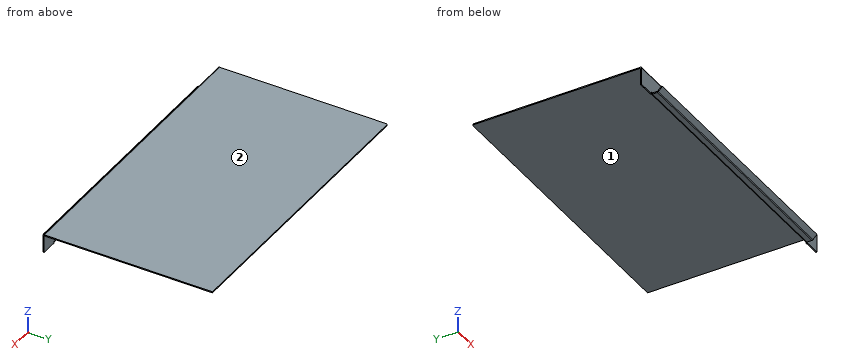
from build123d import *

# Parameters (mm, degrees)
SKETCH_1_W                        = 400
SKETCH_1_H                        = 230
SM_BASE_FLANGE_1_DEPTH            = 1.5
SM_EDGE_FLANGE_1_STRIP_W          = 6.6
SM_EDGE_FLANGE_1_STRIP_H          = 1.5
SM_EDGE_FLANGE_1_STRIP_CUT_DEPTH  = 400
SM_EDGE_FLANGE_1_DEPTH            = 400
SM_EDGE_FLANGE_2_STRIP_W          = 7
SM_EDGE_FLANGE_2_STRIP_H          = 1.5
SM_EDGE_FLANGE_2_STRIP_CUT_DEPTH  = 353
SM_EDGE_FLANGE_2_RELIEF_W         = 7.75
SM_EDGE_FLANGE_2_RELIEF_H         = 0.75
SM_EDGE_FLANGE_2_RELIEF_CUT_DEPTH = 1.5
SM_EDGE_FLANGE_2_DEPTH            = 353
FILLET_1_R                        = 2
SM_START                          = -176.5
SM_EDGE_FLANGE_3_DEPTH            = 353
SM_EDGE_FLANGE_3_2_DEPTH          = 353


# Read off the part's stored shape, not the designer's step: 边线-法兰3
# Sheet-metal steps are written as plain solids
with BuildPart() as part:
    # Sketch 1 → 基体-法兰1 (new body)
    with BuildSketch(Plane.XY):
        Rectangle(SKETCH_1_W, SKETCH_1_H)
    extrude(amount=-SM_BASE_FLANGE_1_DEPTH)

    # 边线-法兰1 strip (across the edge) → 边线-法兰1 strip cut (cut)
    with BuildSketch(Plane(origin=(200, -115, -1.5), x_dir=(0, 1, 0), z_dir=(-1, 0, 0))):
        with Locations((-1.5, -0.75)):
            Rectangle(SM_EDGE_FLANGE_1_STRIP_W, SM_EDGE_FLANGE_1_STRIP_H)
    extrude(amount=SM_EDGE_FLANGE_1_STRIP_CUT_DEPTH, mode=Mode.SUBTRACT)

    # 边线-法兰1 section (across the edge) → 边线-法兰1 (add)
    with BuildSketch(Plane(origin=(200, -115, -1.5), x_dir=(0, 1, 0), z_dir=(-1, 0, 0))):
        with BuildLine():
            Line((0, 0.3), (0, 23.5))
            Line((0, 23.5), (1.5, 23.5))
            Line((1.5, 23.5), (1.5, 0.3))
            ThreePointArc((1.5, 0.3), (1.587867966, 0.087867966), (1.8, 0))
            Line((1.8, 0), (1.8, -1.5))
            ThreePointArc((1.8, -1.5), (0.527207794, -0.972792206), (0, 0.3))
        make_face()
    extrude(amount=SM_EDGE_FLANGE_1_DEPTH)

    # 边线-法兰2 strip (across the edge) → 边线-法兰2 strip cut (cut)
    with BuildSketch(Plane(origin=(-176.5, -115, -25), x_dir=(0, 0, 1), z_dir=(1, 0, 0))):
        with Locations((-1.5, -0.75)):
            Rectangle(SM_EDGE_FLANGE_2_STRIP_W, SM_EDGE_FLANGE_2_STRIP_H)
    extrude(amount=SM_EDGE_FLANGE_2_STRIP_CUT_DEPTH, mode=Mode.SUBTRACT)

    # 边线-法兰2 relief (on the sheet) → 边线-法兰2 relief cut (cut)
    with BuildSketch(Plane(origin=(-176.5, -115, -23), x_dir=(0, 0, 1), z_dir=(0, -1, 0))):
        with Locations((-3.125, 0.375)):
            Rectangle(SM_EDGE_FLANGE_2_RELIEF_W, SM_EDGE_FLANGE_2_RELIEF_H)
        with Locations((-3.125, -353.375)):
            Rectangle(SM_EDGE_FLANGE_2_RELIEF_W, SM_EDGE_FLANGE_2_RELIEF_H)
    extrude(amount=-SM_EDGE_FLANGE_2_RELIEF_CUT_DEPTH, mode=Mode.SUBTRACT)

    # 边线-法兰2 section (across the edge) → 边线-法兰2 (add)
    with BuildSketch(Plane(origin=(-176.5, -115, -25), x_dir=(0, 0, 1), z_dir=(1, 0, 0))):
        with BuildLine():
            Line((0, 0.5), (0, 9.5))
            Line((0, 9.5), (1.5, 9.5))
            Line((1.5, 9.5), (1.5, 0.5))
            ThreePointArc((1.5, 0.5), (1.646446609, 0.146446609), (2, 0))
            Line((2, 0), (2, -1.5))
            ThreePointArc((2, -1.5), (0.585786438, -0.914213562), (0, 0.5))
        make_face()
    extrude(amount=SM_EDGE_FLANGE_2_DEPTH)

    # 圆角1
    fillet_1_edges = [part.edges().sort_by_distance(p)[0] for p in [
        (-200, 115, -0.75),
    ]]
    fillet(fillet_1_edges, radius=FILLET_1_R)

    # 边线-法兰3 outline → 边线-法兰3 (cut)
    with BuildSketch(Plane.YZ.offset(SM_START)):
        with BuildLine():
            ThreePointArc((-122.171572875, -25), (-122.93693974, -24.847759065), (-123.585786438, -24.414213562))
            Line((-123.585786438, -24.414213562), (-124.5, -23.5))
            Line((-124.5, -23.5), (-124.5, -25))
            Line((-124.5, -25), (-122.171572875, -25))
        make_face()
    extrude(amount=SM_EDGE_FLANGE_3_DEPTH, mode=Mode.SUBTRACT)

    # Sm Edge Flange 3 2 outline → Sm Edge Flange 3 2 (add)
    with BuildSketch(Plane.YZ.offset(SM_START)):
        with BuildLine():
            Line((-129.096194078, -18.903805922), (-124.5, -23.5))
            Line((-124.5, -23.5), (-122.171572875, -23.5))
            ThreePointArc((-122.171572875, -23.5), (-122.362914591, -23.461939766), (-122.525126266, -23.353553391))
            Line((-122.525126266, -23.353553391), (-128.035533906, -17.843145751))
            Line((-128.035533906, -17.843145751), (-129.096194078, -18.903805922))
        make_face()
    extrude(amount=SM_EDGE_FLANGE_3_2_DEPTH)


solid = part.part
Design review of the part built by this model. Coordinates are the model's own, in mm. Face numbers are marked on the shaded views. A direction names the side the tool comes from. Round coordinates to 2 decimals unless told otherwise and drop trailing zeros. Write each loop counter-clockwise with the first axis right and the second up, starting at its lowest first coordinate (ties: lowest second). Pieces come first, ordered by that corner, then holes. Notation, with made-up numbers: M 35,-28.5 L 93,-28.5 A19 ccw 93,-4.5 Z; hole C -38,32.5 d7. An arc over 180 degrees is marked long. One line per item, written item: value. Start each with the question number.
1. Clearance check with flat-ended pins moving along their axes: P1, Ø1, axis at x = 81.5, z = -10.5, coming from the +Y side; P2, Ø5.5, axis at y = -124, z = -22, coming from the +X side; P3, Ø5.5, axis at x = 79.5, y = -119, coming from the +Z side; P4, Ø3.5, axis at y = -118, z = -21, coming from the -X side. State where each tip first meets the part, or that it passes through.
2. Take a section at B-B on z = -11.75. State the section outline as (x, y) points.
3. For the marked faces 1 and 2, list the 3-axis set-ups (+Z, -Z, +X, -X, +Y, -Y) from which the entire face can be reached by the end or side of a thin tool; tool diameter is ignored.
4. Take a section at A-A on x = -78. State the section outline as (y, z) points, then the cut area to 3 significant figures.
5. Take a section at C-C on y = -15.5. State the section outline as (x, z) points, then the cut area to 3 significant figures.
6. To check wall thickness, follow probe 1 along Z at (x, y) = (-176, 7); probe 2 along Y at (x, z) = (173.5, -14.5); probe 3 along Y at (x, z) = (36, -19). State the ranges of each line that lie inside material, in increasing order. Write a range as from..to.
Computed:
1. P1: stops at y = -113.5
1. P2: stops at x = 176.5
1. P3: stops at z = -23.5
1. P4: passes through
2. outline: M -200,-115 L 200,-115 L 200,-113.5 L -200,-113.5 Z
3. face 1: -Z, +X, -X, +Y
3. face 2: +Z, +X, -X, +Y, -Y
4. outline: M -129.1,-18.9 L -123.59,-24.41 A2 ccw -122.17,-25 L -115.5,-25 A2 ccw -113.5,-23 L -113.5,-1.8 A0.3 cw -113.2,-1.5 L 115,-1.5 L 115,0 L -113.2,0 A1.8 ccw -115,-1.8 L -115,-23 A0.5 cw -115.5,-23.5 L -122.17,-23.5 A0.5 cw -122.53,-23.35 L -128.04,-17.84 Z
4. area: 403 mm²
5. outline: M -200,-1.5 L 200,-1.5 L 200,0 L -200,0 Z
5. area: 600 mm²
6. probe 1: z = -1.5..0
6. probe 2: y = -115..-113.5
6. probe 3: y = -129..-126.88, -115..-113.5
